Source: CAD feature listing. Evaluate the final solid. Frame: model axes, mm. Round coordinates to 2 decimals unless told otherwise and drop trailing zeros. Loops run counter-clockwise (first coordinate to the right, second up) from the corner with the lowest first, then second, coordinate; pieces in that order, holes last.
Item 1: Section query C-C on x = 132.5. Return loops of the section in (y, z).
Item 2: Section query D-D on z = 1.2. Give the number of separate pieces and of enclosed holes in the cut face, then the cut area to 3 significant figures.
Item 3: Section query B-B on x = 26.5. Return loops of the section in (y, z), then the cut area to 3 significant figures.
Item 4: Ray query, L1, parallel to Y at x = 95, z = 1.5; L2, parallel to X at y = 6, z = 0.45; L3, parallel to Y at x = 214, z = 2.75. Return the intervals inside material, ascending.
Item 5: Section query A-A on y = 85. Return loops of the section in (x, z).
Autodesk Inventor part; units mm, degrees
ref_plane "YZ Plane" through (0, 0, 0) normal (1, 0, 0) x (0, 1, 0)
ref_plane "XZ Plane" through (0, 0, 0) normal (0, 1, 0) x (-1, 0, 0)
ref_plane "XY Plane" through (0, 0, 0) normal (0, 0, 1) x (1, 0, 0)
sketch "Sketch1" plane through (0, 0, 0) normal (0, 0, 1) x (1, 0, 0)
  line L0 (0, 0) -> (20, 0)
  line L1 (0, 0) -> (0, -5)
  line L2 (20, -5) -> (0, -5)
  line L3 (20, 0) -> (20, -5)
  line L4 (76, 0) -> (76, -5)
  line L5 (76, 0) -> (136, 0)
  line L6 (136, -5) -> (76, -5)
  line L7 (136, 0) -> (136, -5)
  line L8 (192, 0) -> (192, -5)
  line L9 (212, 0) -> (192, 0)
  line L10 (212, -5) -> (192, -5)
  line L11 (212, 0) -> (212, -5)
  line L12 (10, -55) -> (10, -60)
  line L13 (30, -55) -> (10, -55)
  line L14 (30, -60) -> (10, -60)
  line L15 (30, -55) -> (30, -60)
  line L16 (76, -55) -> (76, -60)
  line L17 (76, -55) -> (136, -55)
  line L18 (136, -60) -> (76, -60)
  line L19 (136, -55) -> (136, -60)
  line L20 (182, -55) -> (182, -60)
  line L21 (182, -55) -> (202, -55)
  line L22 (202, -60) -> (182, -60)
  line L23 (202, -55) -> (202, -60)
  line L24 (236, -70.0001) -> (236, -80.0001) construction
  line L25 (239.5, -70.0001) -> (236, -70.0001) construction
  line L26 (239.5, -70.0001) -> (239.5, -80.0001) construction
  line L27 (236, -80.0001) -> (239.5, -80.0001) construction
  line L28 (-27.5, -80) -> (-27.5, -70) construction
  line L29 (-24, -70) -> (-27.5, -70) construction
  line L30 (-24, -70) -> (-24, -80) construction
  line L31 (-24, -80) -> (-27.5, -80) construction
  line L32 (-27.5, -60) -> (-27.5, -20)
  line L33 (-24, -20) -> (-27.5, -20)
  line L34 (-24, -60) -> (-24, -20)
  line L35 (-24, -60) -> (-27.5, -60)
  line L36 (-27.5, 0) -> (-27.5, 40)
  line L37 (-24, 40) -> (-24, 0)
  line L38 (-24, 40) -> (-27.5, 40)
  line L39 (-24, 0) -> (-27.5, 0)
  line L40 (-27.5, 60) -> (-27.5, 100)
  line L41 (-24, 100) -> (-27.5, 100)
  line L42 (-24, 100) -> (-24, 60)
  line L43 (-24, 60) -> (-27.5, 60)
  line L44 (-27.5, 160) -> (-27.5, 120)
  line L45 (-24, 160) -> (-24, 120)
  line L46 (-24, 160) -> (-27.5, 160)
  line L47 (236, -0.0001) -> (236, 39.9999)
  line L48 (239.5, 39.9999) -> (239.5, -0.0001)
  line L49 (239.5, 39.9999) -> (236, 39.9999)
  line L50 (239.5, -0.0001) -> (236, -0.0001)
  line L51 (236, -60.0001) -> (236, -20.0001)
  line L52 (239.5, -60.0001) -> (239.5, -20.0001)
  line L53 (239.5, -20.0001) -> (236, -20.0001)
  line L54 (239.5, -60.0001) -> (236, -60.0001)
  line L55 (239.5, 99.9999) -> (236, 99.9999)
  line L56 (236, 59.9999) -> (236, 99.9999)
  line L57 (239.5, 99.9999) -> (239.5, 59.9999)
  line L58 (239.5, 59.9999) -> (236, 59.9999)
  line L59 (236, 159.9999) -> (236, 119.9999)
  line L60 (239.5, 159.9999) -> (239.5, 119.9999)
  line L61 (236, 159.9999) -> (239.5, 159.9999)
  line L62 (236, 111.9999) -> (239.5, 111.9999) construction
  line L63 (239.5, 107.9999) -> (236, 107.9999) construction
  line L64 (236, 51.9999) -> (239.5, 51.9999) construction
  line L65 (239.5, 47.9999) -> (236, 47.9999) construction
  line L66 (236, -66.0001) -> (239.5, -66.0001) construction
  line L67 (212, -60) -> (212, -55) construction
  line L68 (216, -55) -> (216, -60) construction
  line L69 (168, -60) -> (168, -55) construction
  line L70 (172, -55) -> (172, -60) construction
  line L71 (40, -60) -> (40, -55) construction
  line L72 (44, -55) -> (44, -60) construction
  line L73 (-4, -60) -> (-4, -55) construction
  line L74 (0, -55) -> (0, -60) construction
  line L75 (-14, -5) -> (-14, 0) construction
  line L76 (-10, 0) -> (-10, -5) construction
  line L77 (30, -5) -> (30, 0) construction
  line L78 (34, 0) -> (34, -5) construction
  line L79 (178, -5) -> (178, 0) construction
  line L80 (182, 0) -> (182, -5) construction
  line L81 (222, -5) -> (222, 0) construction
  line L82 (226, 0) -> (226, -5) construction
  line L83 (-27.5, -66) -> (-24, -66) construction
  line L84 (-27.5, 52) -> (-24, 52) construction
  line L85 (-24, 48) -> (-27.5, 48) construction
  line L86 (-24, 108) -> (-27.5, 108) construction
  line L87 (-27.5, 112) -> (-24, 112) construction
  line L88 (-24, 120) -> (-27.5, 120)
  line L89 (239.5, 119.9999) -> (236, 119.9999)
  line L90 (-25.75, 112) -> (-25.75, 108) construction
  circle A0 centre (-25.75, 110) radius 2
  line L91 (-25.75, 52) -> (-25.75, 48) construction
  circle A1 centre (-25.75, 50) radius 2
  line L92 (-25.75, -66) -> (-25.75, -70) construction
  circle A2 centre (-25.75, -68) radius 2
  line L93 (237.75, 111.9999) -> (237.75, 107.9999) construction
  circle A3 centre (237.75, 109.9999) radius 2
  line L94 (237.75, 51.9999) -> (237.75, 47.9999) construction
  circle A4 centre (237.75, 49.9999) radius 2
  line L95 (237.75, -66.0001) -> (237.75, -70.0001) construction
  circle A5 centre (237.75, -68.0001) radius 2
  line L96 (-14, -2.5) -> (-10, -2.5) construction
  line L97 (30, -2.5) -> (34, -2.5) construction
  line L98 (178, -2.5) -> (182, -2.5) construction
  line L99 (222, -2.5) -> (226, -2.5) construction
  line L100 (212, -57.5) -> (216, -57.5) construction
  line L101 (168, -57.5) -> (172, -57.5) construction
  line L102 (40, -57.5) -> (44, -57.5) construction
  line L103 (-4, -57.5) -> (0, -57.5) construction
  circle A6 centre (-12, -2.5) radius 2
  circle A7 centre (32, -2.5) radius 2
  circle A8 centre (180, -2.5) radius 2
  circle A9 centre (224, -2.5) radius 2
  circle A10 centre (214, -57.5) radius 2
  circle A11 centre (170, -57.5) radius 2
  circle A12 centre (42, -57.5) radius 2
  circle A13 centre (-2, -57.5) radius 2
  line L104 (-27.5, -80) -> (-42.5, -80) construction
  line L105 (239.5, 159.9999) -> (254.5, 159.9999) construction
  line L106 (254.5, 159.9999) -> (254.5, 179.9999) construction
  line L107 (254.5, 179.9999) -> (239.5, 179.9999) construction
  line L108 (239.5, 179.9999) -> (239.5, 159.9999) construction
  line L109 (254.5, 179.9999) -> (-42.5, 179.9999)
  line L110 (-42.5, 179.9999) -> (-42.5, -80)
  line L111 (-42.5, -80) -> (254.5, -80)
  line L112 (254.5, -80) -> (254.5, 179.9999)
  dimension "d0" = 15
  dimension "d3" = 15
  dimension "d4" = 20
extrude "Extrusion1" add sketch "Sketch1" along normal blind 3.5
fillet "Fillet1" radius 8 4 edges at (254.5, 179.9999, 1.75) (-42.5, 179.9999, 1.75) (254.5, -80, 1.75) (-42.5, -80, 1.75)
sketch "Sketch2" plane through (0, 0, 3.5) normal (0, 0, 1) x (1, 0, 0)
  arc A0 (-42.5, -72) -> (-34.5, -80) centre (-34.5, -72) ccw construction
  line L0 (-34.5, -80) -> (246.5, -80) construction
  arc A1 (246.5, -80) -> (254.5, -72) centre (246.5, -72) ccw construction
  line L1 (254.5, -72) -> (254.5, 171.9999) construction
  arc A2 (254.5, 171.9999) -> (246.5, 179.9999) centre (246.5, 171.9999) ccw construction
  line L2 (246.5, 179.9999) -> (-34.5, 179.9999) construction
  arc A3 (-34.5, 179.9999) -> (-42.5, 171.9999) centre (-34.5, 171.9999) ccw construction
  line L3 (-42.5, 171.9999) -> (-42.5, -72) construction
  line L4 (76, -55) -> (136, -55) construction
  line L5 (136, -55) -> (136, -60) construction
  line L6 (136, -60) -> (76, -60) construction
  line L7 (76, -60) -> (76, -55) construction
  line L8 (76, 0) -> (136, 0) construction
  line L9 (136, 0) -> (136, -5) construction
  line L10 (136, -5) -> (76, -5) construction
  line L11 (76, -5) -> (76, 0) construction
  line L12 (236, 159.9999) -> (239.5, 159.9999) construction
  line L13 (239.5, 159.9999) -> (239.5, 119.9999) construction
  line L14 (239.5, 119.9999) -> (236, 119.9999) construction
  line L15 (236, 119.9999) -> (236, 159.9999) construction
  line L16 (239.5, 99.9999) -> (239.5, 59.9999) construction
  line L17 (239.5, 59.9999) -> (236, 59.9999) construction
  line L18 (236, 59.9999) -> (236, 99.9999) construction
  line L19 (236, 99.9999) -> (239.5, 99.9999) construction
  line L20 (236, -20.0001) -> (239.5, -20.0001) construction
  line L21 (239.5, -20.0001) -> (239.5, -60.0001) construction
  line L22 (239.5, -60.0001) -> (236, -60.0001) construction
  line L23 (236, -60.0001) -> (236, -20.0001) construction
  line L24 (236, 39.9999) -> (239.5, 39.9999) construction
  line L25 (239.5, 39.9999) -> (239.5, -0.0001) construction
  line L26 (239.5, -0.0001) -> (236, -0.0001) construction
  line L27 (236, -0.0001) -> (236, 39.9999) construction
  line L28 (-27.5, 160) -> (-24, 160) construction
  line L29 (-24, 160) -> (-24, 120) construction
  line L30 (-24, 120) -> (-27.5, 120) construction
  line L31 (-27.5, 120) -> (-27.5, 160) construction
  line L32 (-27.5, 100) -> (-24, 100) construction
  line L33 (-24, 100) -> (-24, 60) construction
  line L34 (-24, 60) -> (-27.5, 60) construction
  line L35 (-27.5, 60) -> (-27.5, 100) construction
  line L36 (-27.5, 40) -> (-24, 40) construction
  line L37 (-24, 40) -> (-24, 0) construction
  line L38 (-24, 0) -> (-27.5, 0) construction
  line L39 (-27.5, 0) -> (-27.5, 40) construction
  line L40 (-27.5, -20) -> (-24, -20) construction
  line L41 (-24, -20) -> (-24, -60) construction
  line L42 (-24, -60) -> (-27.5, -60) construction
  line L43 (-27.5, -60) -> (-27.5, -20) construction
  line L44 (182, -55) -> (202, -55) construction
  line L45 (202, -55) -> (202, -60) construction
  line L46 (202, -60) -> (182, -60) construction
  line L47 (182, -60) -> (182, -55) construction
  line L48 (10, -55) -> (30, -55) construction
  line L49 (30, -55) -> (30, -60) construction
  line L50 (30, -60) -> (10, -60) construction
  line L51 (10, -60) -> (10, -55) construction
  line L52 (192, 0) -> (212, 0) construction
  line L53 (212, 0) -> (212, -5) construction
  line L54 (212, -5) -> (192, -5) construction
  line L55 (192, -5) -> (192, 0) construction
  line L56 (20, 0) -> (20, -5) construction
  line L57 (20, -5) -> (0, -5) construction
  line L58 (0, -5) -> (0, 0) construction
  line L59 (0, 0) -> (20, 0) construction
  circle A4 centre (-2, -57.5) radius 2 construction
  circle A5 centre (42, -57.5) radius 2 construction
  circle A6 centre (170, -57.5) radius 2 construction
  circle A7 centre (214, -57.5) radius 2 construction
  circle A8 centre (224, -2.5) radius 2 construction
  circle A9 centre (180, -2.5) radius 2 construction
  circle A10 centre (32, -2.5) radius 2 construction
  circle A11 centre (-12, -2.5) radius 2 construction
  circle A12 centre (237.75, -68.0001) radius 2 construction
  circle A13 centre (237.75, 49.9999) radius 2 construction
  circle A14 centre (237.75, 109.9999) radius 2 construction
  circle A15 centre (-25.75, -68) radius 2 construction
  circle A16 centre (-25.75, 50) radius 2 construction
  circle A17 centre (-25.75, 110) radius 2 construction
  line L60 (-24, 160) -> (236, 159.9999) construction
  line L61 (-19, 160) -> (231, 160)
  line L62 (231, 160) -> (231, 163.5)
  line L63 (231, 163.5) -> (-19, 163.5)
  line L64 (-19, 163.5) -> (-19, 160)
  dimension "d8" = 250
  dimension "d9" = 3.5
  dimension "d10" = 5
extrude "Extrusion2" cut sketch "Sketch2" against normal blind 3.5
properties part number "Tapa_Frontal"
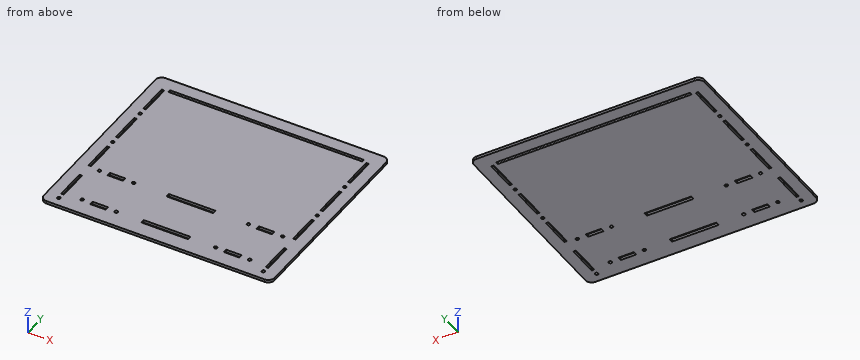
Data:
1. outline: (-80, 0) - (-60, 0) - (-60, 3.5) - (-80, 3.5) - close; (-55, 0) - (-5, 0) - (-5, 3.5) - (-55, 3.5) - close; (0, 0) - (160, 0) - (160, 3.5) - (0, 3.5) - close; (163.5, 0) - (180, 0) - (180, 3.5) - (163.5, 3.5) - close
2. separate pieces: 1
2. enclosed holes: 29
2. area: 74,000 mm2
3. outline: (-80, 0) - (-60, 0) - (-60, 3.5) - (-80, 3.5) - close; (-55, 0) - (160, 0) - (160, 3.5) - (-55, 3.5) - close; (163.5, 0) - (180, 0) - (180, 3.5) - (163.5, 3.5) - close
3. area: 880 mm2
4. L1: y = -80 to -60, -55 to -5, 0 to 160, 163.5 to 180
4. L2: x = -42.5 to -27.5, -24 to 236, 239.5 to 254.5
4. L3: y = -80 to -59.5, -55.5 to 160, 163.5 to 180
5. outline: (-42.5, 0) - (-27.5, 0) - (-27.5, 3.5) - (-42.5, 3.5) - close; (-24, 0) - (236, 0) - (236, 3.5) - (-24, 3.5) - close; (239.5, 0) - (254.5, 0) - (254.5, 3.5) - (239.5, 3.5) - close
